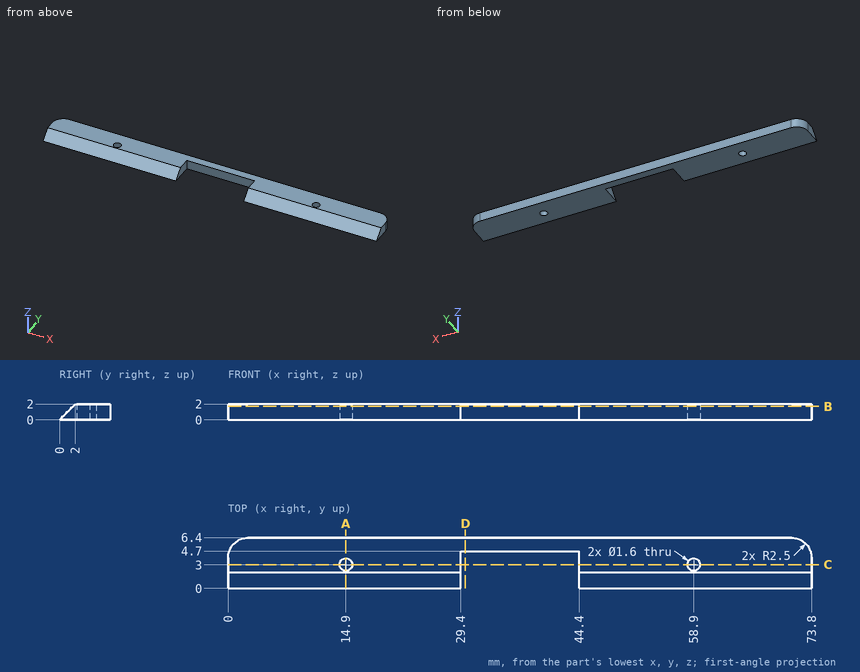
Part print with two shaded views. Sizes in mm from the minimum x, y, z corner. Coordinates: 2 decimals unless noted, no trailing zeros. Order: outer loops, then holes, each group sorted by start corner. A loop starts at its lowest first (then second) coordinate and runs counter-clockwise, first axis right, second up. Notation, with made-up numbers: M 32,43 L 56,43 A22 ccw 56,61 Z; hole C 56,-21 d9. An arc over 180 degrees is marked long. One line per question, with ' | ' between items. Start each with the question number.
1. Cut at C-C (y = 3). Write the cut outline in (x, z), plus the area to 3 significant figures.
2. Wall check: line 1 along X through (y, z) = (1.75, 0.2); line 2 along Y through (x, z) = (41, 0.45); line 3 along X through (y, z) = (3.5, 0.4). Give the ranges that are in metal, low to high. Write a range as [from, to].
3. Cut at B-B (z = 1.7). Write the cut outline in (x, y).
4. Flat gauge pins, fed straight in: P1, Ø1.3, axis at x = 58.9, y = 3, coming from the -Z side; P2, Ø0.6, axis at x = 38, z = 0.5, coming from the -Y side; P3, Ø1, axis at y = 5.5, z = 1, coming from the +X side (3 decimals). Where does each tip first touch, or does it go through?
5. Cut at D-D (x = 30). Write the cut outline in (y, z).
6. Cut at A-A (x = 14.9). Write the cut outline in (y, z).
The answers:
1) outline: M 0,0 L 14.1,0 L 14.1,2 L 0,2 Z; M 15.7,0 L 29.4,0 L 29.4,2 L 15.7,2 Z; M 44.4,0 L 58.1,0 L 58.1,2 L 44.4,2 Z; M 59.7,0 L 73.8,0 L 73.8,2 L 59.7,2 Z | area: 111 mm2
2) line 1: x = [0, 29.4], [44.4, 73.8] | line 2: y = [4.7, 6.4] | line 3: x = [0, 14.28], [15.52, 29.4], [44.4, 58.28], [59.52, 73.8]
3) outline: M 0,1.7 L 29.4,1.7 L 29.4,4.7 L 44.4,4.7 L 44.4,1.7 L 73.8,1.7 L 73.8,3.9 A2.5 ccw 71.3,6.4 L 2.5,6.4 A2.5 ccw 0,3.9 Z; hole C 14.9,3 d1.6; hole C 58.9,3 d1.6
4) P1: passes through | P2: stops at y = 4.7 | P3: stops at x = 73.545
5) outline: M 4.7,0 L 6.4,0 L 6.4,2 L 4.7,2 Z
6) outline: M 0,0 L 2.2,0 L 2.2,2 L 2,2 Z; M 3.8,0 L 6.4,0 L 6.4,2 L 3.8,2 Z
